from build123d import *

# Parameters (mm, degrees)
OUTER_BLOCK_SKETCH_W               = 30
OUTER_BLOCK_SKETCH_H               = 20
MAIN_BLOCK_DEPTH                   = 5
BELT_TRAP_BLOCK_SKETCH_W           = 5.9
BELT_TRAP_BLOCK_SKETCH_H           = 20
BELT_TRAP_BLOCK_DEPTH              = 5
M3_CLEARANCE_HOLE1_D               = 3.4
BELT_TRAPPING_RIDGE_MASTER_DEPTH   = 5.9
BELT_TRAPPING_RIDGES_PATTERN_COUNT = 10
BELT_TRAPPING_RIDGES_PATTERN_PITCH = 2
PRINT_HELPER_FILLETS_R             = 1


with BuildPart() as part:
    # Outer Block Sketch → Main Block (new body)
    with BuildSketch(Plane.XY):
        Rectangle(OUTER_BLOCK_SKETCH_W, OUTER_BLOCK_SKETCH_H)
    extrude(amount=MAIN_BLOCK_DEPTH)

    # Belt Trap Block Sketch → Belt Trap Block (add)
    with BuildSketch(Plane.XY):
        Rectangle(BELT_TRAP_BLOCK_SKETCH_W, BELT_TRAP_BLOCK_SKETCH_H)
    extrude(amount=-BELT_TRAP_BLOCK_DEPTH)

    # M3 Clearance Hole1 (through all)
    with Locations(Plane.XY.offset(5)):
        with Locations((-10, 5), (10, 5), (-10, -5), (10, -5)):
            Hole(M3_CLEARANCE_HOLE1_D / 2)

    # Belt Trapping Ridges Sketch → Belt Trapping Ridge (Master) (add)
    with BuildSketch(Plane(origin=(2.95, 0, 0), x_dir=(0, 0, -1), z_dir=(1, 0, 0))):
        with BuildLine():
            Line((5, 10), (5.1, 10))
            ThreePointArc((5.1, 10), (5.6, 9.5), (5.1, 9))
            Line((5.1, 9), (5, 9))
            Line((5, 9), (5, 10))
        make_face()
    belt_trapping_ridge_master = extrude(amount=-BELT_TRAPPING_RIDGE_MASTER_DEPTH)

    # Belt Trapping Ridges Pattern: Belt Trapping Ridge (Master) ×10
    with Locations(*[(0, -i * BELT_TRAPPING_RIDGES_PATTERN_PITCH, 0) for i in range(1, BELT_TRAPPING_RIDGES_PATTERN_COUNT)]):
        add(belt_trapping_ridge_master)

    # Print Helper Fillets
    print_helper_fillets_edges = [part.edges().sort_by_distance(p)[0] for p in [
        (15, -10, 2.5),
        (15, 10, 2.5),
        (-15, -10, 2.5),
        (-15, 10, 2.5),
        (-2.95, -10, -2.5),
        (2.95, -10, -2.5),
    ]]
    fillet(print_helper_fillets_edges, radius=PRINT_HELPER_FILLETS_R)


solid = part.part
Can you work these out from the model? Positions are in its coordinate system, mm. A direction names the side the tool comes from. Give positions to 0.01 mm unless a question says otherwise; leave off trailing zeros. Order: outer loops, then holes, each group sorted by start corner. A loop starts at its lowest first (then second) coordinate and runs counter-clockwise, first axis right, second up. Notation, with made-up numbers: M 82.5,37 L 107.5,37 A13 cw 107.5,56 Z; hole C 30.25,22 d4. An arc over 180 degrees is marked long. One line per question, with ' | ' between items.
Item 1: Suppose I cut it at B-B, the plane z = 2.75. Write out the boundary of the cut face in (x, y).
Answer block:
outline: M -15,-9 A1 ccw -14,-10 L 14,-10 A1 ccw 15,-9 L 15,9 A1 ccw 14,10 L -14,10 A1 ccw -15,9 Z; hole C -10,-5 d3.4; hole C -10,5 d3.4; hole C 10,-5 d3.4; hole C 10,5 d3.4
Item 2: For faces 4 (the face through (-2.665, -9.699, -2.535)), 5 (the face through (0, -9.5, -5)), 6 (the face through (-2.95, 1, -3)), which set-ups out of +Z, -Z, +X, -X, +Y, -Y let a thin tool reach every point of the face, with its end or its side?
Answer block:
face 4: -Z, -X, -Y | face 5: -Z, +X, -X, -Y | face 6: -Z, -X, +Y, -Y
Item 3: Please list where these lines run through material, in increasing order: L1, parallel to Y at x = 10, z = 2; L2, parallel to X at y = 6.25, z = 0.25; L3, parallel to X at y = 3.5, z = 2.75.
Answer block:
L1: y = -10 to -6.7, -3.3 to 3.3, 6.7 to 10 | L2: x = -15 to -11.15, -8.85 to 8.85, 11.15 to 15 | L3: x = -15 to -10.8, -9.2 to 9.2, 10.8 to 15
Item 4: Suppose I cut it at C-C, the plane y = 7.5. Write out the boundary of the cut face in (x, z), then the cut area to 3 significant figures.
Answer block:
outline: M -15,0 L -2.95,0 L -2.95,-5.6 L 2.95,-5.6 L 2.95,0 L 15,0 L 15,5 L -15,5 Z | area: 183 mm2
Item 5: Suppose I cut it at D-D, the plane y = 5.5. Write out the boundary of the cut face in (x, z), then the cut area to 3 significant figures.
Answer block:
outline: M -15,0 L -11.62,0 L -11.62,5 L -15,5 Z; M -8.38,0 L -2.95,0 L -2.95,-5.6 L 2.95,-5.6 L 2.95,0 L 8.38,0 L 8.38,5 L -8.38,5 Z; M 11.62,0 L 15,0 L 15,5 L 11.62,5 Z | area: 151 mm2
Item 6: Suppose I cut it at A-A, the plane x = 10. Write out the boundary of the cut face in (y, z).
Answer block:
outline: M -10,0 L -6.7,0 L -6.7,5 L -10,5 Z; M -3.3,0 L 3.3,0 L 3.3,5 L -3.3,5 Z; M 6.7,0 L 10,0 L 10,5 L 6.7,5 Z
Item 7: I'm going to push flat-ended pins straight in: pin 1 Ø0.5 at (x, y) = (1.5, 6.5) entering from -Z; pin 2 Ø2 at (x, y) = (-8.5, 3) entering from -Z; pin 3 Ø2 at (y, z) = (-1.5, -3) entering from -X. Where does each tip first touch, or does it pass through?
Answer block:
pin 1: stops at z = -5 | pin 2: stops at z = 0 | pin 3: stops at x = -2.95
Item 8: We'd pull the mould along Y, two halves only. Please class faces 1 (the face through (14.699, 9.715, 2.535)), 2 (the face through (0, 0, 5)), 3 (the face through (0, -1.5, -5)): released by +Y, released by -Y, zero draft, split by the parting line, or undercut.
Answer block:
face 1: released by +Y | face 2: zero draft | face 3: undercut
